Input: part model. Units: mm. Frame: model coordinates. A direction names the side the tool comes from. Give positions to 0.01 mm unless a question says otherwise; leave off trailing zeros. Loops run counter-clockwise (first coordinate to the right, second up) from the corner with the lowest first, then second, coordinate; pieces in that order, holes last. Notation, with made-up numbers: (53, 37.25) - (85, 37.25) arc R16 cw to (85, 59.25) - close; hole circle Ø10 at (73.5, -1.5). An arc over 180 degrees is marked (long way). Answer as a JSON object with one key per item and string values.
from build123d import *

# Parameters (mm, degrees)
SKETCH_1_R          = 4
EXTRUDE_1_DEPTH     = 10
SKETCH_2_R          = 2
EXTRUDE_2_DEPTH     = 8
SKETCH_3_R          = 3
EXTRUDE_3_DEPTH     = 16
EXTRUDE_START       = 8
SKETCH_4_R          = 2
EXTRUDE_4_DEPTH     = 8
CHAMFER_1_SIZE      = 1
CUT_EXTRUDE_START   = -10
SKETCH_5_R          = 3
SKETCH_5_R_2        = 2.5
CUT_EXTRUDE_1_DEPTH = 10


with BuildPart() as part:
    # 草图1 → 凸台-拉伸1 (new body)
    with BuildSketch(Plane(origin=(0, 0, 0), x_dir=(0, 0, -1), z_dir=(1, 0, 0))):
        Circle(SKETCH_1_R)
    extrude(amount=EXTRUDE_1_DEPTH)

    # 草图2 → 凸台-拉伸2 (add)
    with BuildSketch(Plane.ZY):
        with Locations(Location((0, 0, 0), (0, 0, 180))):
            Circle(SKETCH_2_R)
    extrude(amount=EXTRUDE_2_DEPTH)

    # 草图3 → 凸台-拉伸3 (add)
    with BuildSketch(Plane(origin=(10, 0, 0), x_dir=(0, 0, -1), z_dir=(1, 0, 0))):
        Circle(SKETCH_3_R)
    extrude(amount=EXTRUDE_3_DEPTH)

    # 草图4 → 凸台-拉伸4 (add)
    with BuildSketch(Plane(origin=(26, 0, 0), x_dir=(0, 0, -1), z_dir=(1, 0, 0)).offset(EXTRUDE_START)):
        Circle(SKETCH_4_R)
    extrude(amount=-EXTRUDE_4_DEPTH)

    # 倒角1
    chamfer_1_edges = [part.edges().sort_by_distance(p)[0] for p in [
        (0, 0, 4),
    ]]
    chamfer(chamfer_1_edges, length=CHAMFER_1_SIZE)

    # 草图5 → 切除-拉伸1 (cut)
    with BuildSketch(Plane(origin=(26, 0, 0), x_dir=(0, 0, -1), z_dir=(1, 0, 0)).offset(CUT_EXTRUDE_START)):
        Circle(SKETCH_5_R)
        Circle(SKETCH_5_R_2, mode=Mode.SUBTRACT)
    extrude(amount=CUT_EXTRUDE_1_DEPTH, mode=Mode.SUBTRACT)


solid = part.part
Item 1: Cut plane C-C (x = 28). Return loops of the section in (y, z).
Geometry check:
{"outline": "circle Ø4 at (0, 0)"}
Item 2: Cut plane D-D (x = 9.5). Return loops of the section in (y, z), then the cut area to 3 significant figures.
Geometry check:
{"outline": "circle Ø8 at (0, 0)", "area": "50.3 mm2"}
Item 3: Access query for faces 1 (the face through (20.93, -2.44, 0.54)), 2 (the face through (5.437, -3.905, 0.867)), 3 (the face through (0, -2, -1)). Directions: +Z, -Z, +X, -X, +Y, -Y. A direction counts if a zero-diameter tool reaches every point of the face in a straight line with its end or side. Return the directions, or none.
Geometry check:
{"face 1": "+X", "face 2": "+X, -X", "face 3": "-X"}
Item 4: Material intervals for line 1 (X direction, y = -2.25, z = -1); line 2 (X direction, y = -0.25, z = 2.75); line 3 (Z direction, x = 24, y = -1.5), sorted ascending. Write a range as [from, to].
Geometry check:
{"line 1": "x = [0, 26]", "line 2": "x = [0, 16]", "line 3": "z = [-2, 2]"}
Item 5: Contact query for flat-ended pins moving along their axis: P1, Ø1, axis at x = -3.5, y = 2, coming from the +Z side; P2, Ø1.5, axis at x = 21.5, y = 2.5, coming from the -Z side; P3, Ø4, axis at x = 16, z = 0.5, coming from the -Y side. Output: stop coordinate, or through.
Geometry check:
{"P1": "stops at z = 1.32", "P2": "stops at z = -1.79", "P3": "stops at y = -3"}
Item 6: Cut plane A-A (y = 0). Return loops of the section in (x, z), then the cut area to 3 significant figures.
Geometry check:
{"outline": "(-8, -2) - (0, -2) - (0, -3) - (1, -4) - (10, -4) - (10, -3) - (16, -3) - (16, -2.5) - (26, -2.5) - (26, -2) - (34, -2) - (34, 2) - (26, 2) - (26, 2.5) - (16, 2.5) - (16, 3) - (10, 3) - (10, 4) - (1, 4) - (0, 3) - (0, 2) - (-8, 2) - close", "area": "229 mm2"}
